Here's the drawing with two shaded views (mm, measured from the low corner). I have some questions. Round coordinates to 2 decimals unless told otherwise and drop trailing zeros. Loops run counter-clockwise (first coordinate to the right, second up) from the corner with the lowest first, then second, coordinate; pieces in that order, holes last. Notation, with made-up numbers: (18.5, -39.75) - (23.5, -39.75) arc R30 cw to (23.5, -3.75) - close; hole circle Ø6 at (70.25, 17). An arc over 180 degrees is marked (long way). Answer as CSV lines item,"result".
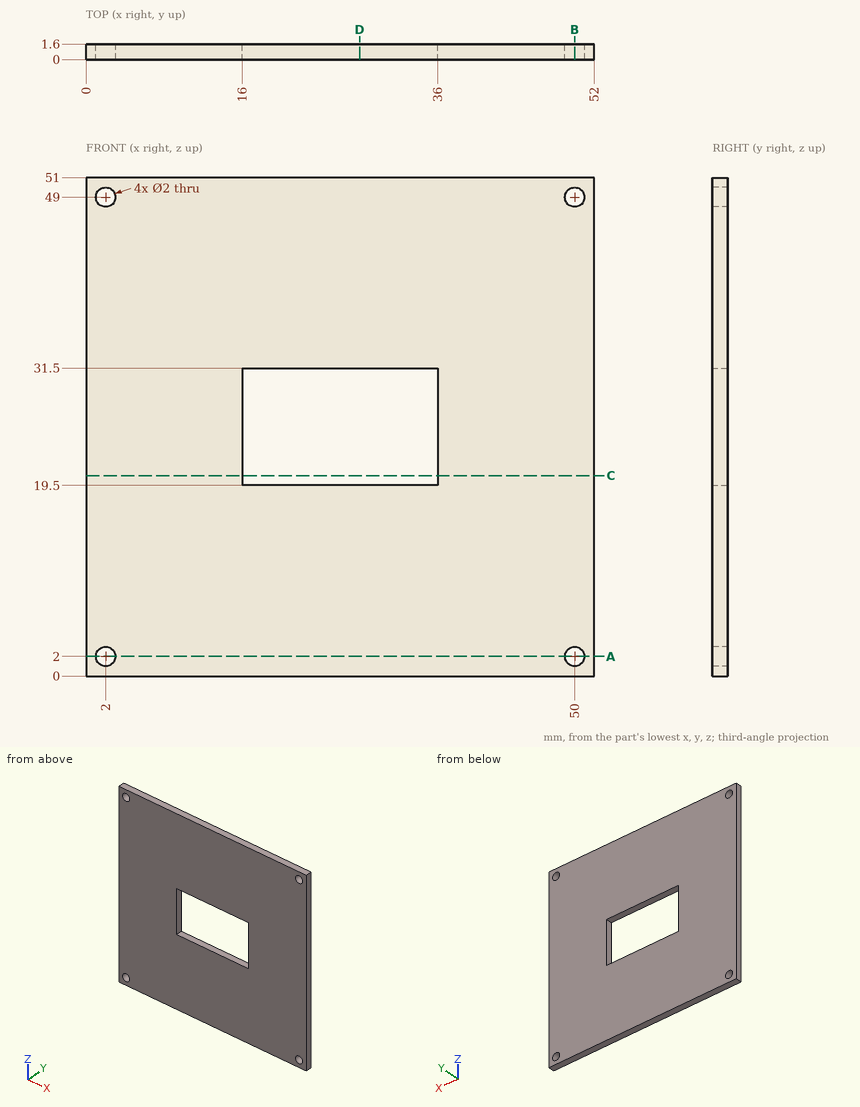
Q1. If I drill on line 1 along Z through (x, y) = (2, 1.3); line 2 along X through (y, z) = (1.5, 48.5); line 3 along X through (y, z) = (1.55, 25.5), over which ranges is the centre line in solid material (lowest first)? Write a range as [from, to].
Checks:
line 1,"[0, 1], [3, 48], [50, 51]"
line 2,"[0, 1.13], [2.87, 49.13], [50.87, 52]"
line 3,"[0, 16], [36, 52]"
Q2. Imagine slicing it at C-C (z = 20.5). Write out the boundary of the cut face in (x, y).
Checks:
outline,"(0, 0) - (16, 0) - (16, 1.6) - (0, 1.6) - close; (36, 0) - (52, 0) - (52, 1.6) - (36, 1.6) - close"
Q3. Imagine slicing it at A-A (z = 2). Write out the boundary of the cut face in (x, y).
Checks:
outline,"(0, 0) - (1, 0) - (1, 1.6) - (0, 1.6) - close; (3, 0) - (49, 0) - (49, 1.6) - (3, 1.6) - close; (51, 0) - (52, 0) - (52, 1.6) - (51, 1.6) - close"
Q4. Imagine slicing it at B-B (x = 50). Write out the boundary of the cut face in (y, z), then the cut area to 3 significant figures.
Checks:
outline,"(0, 0) - (1.6, 0) - (1.6, 1) - (0, 1) - close; (0, 3) - (1.6, 3) - (1.6, 48) - (0, 48) - close; (0, 50) - (1.6, 50) - (1.6, 51) - (0, 51) - close"
area,"75.2 mm²"
Q5. Imagine slicing it at D-D (x = 28). Write out the boundary of the cut face in (y, z), then the cut area to 3 significant figures.
Checks:
outline,"(0, 0) - (1.6, 0) - (1.6, 19.5) - (0, 19.5) - close; (0, 31.5) - (1.6, 31.5) - (1.6, 51) - (0, 51) - close"
area,"62.4 mm²"
Q6. I'm going to push a flat-ended pin straight in: pin 1 Ø0.5 at (x, y) = (23.5, 1) entering from -Z. Where does the tip first touch, or does it pass through?
Checks:
pin 1,"z = 0"
